from build123d import *

# Parameters (mm, degrees)
BOSS_EXTRUDE2_DEPTH = 5
SKETCH8_R           = 50
CUT_EXTRUDE6_DEPTH  = 20
SKETCH9_OUTSIDE_W   = 10.721
SKETCH9_OUTSIDE_H   = 17.86
SKETCH9_OUTSIDE_R   = 50
CUT_EXTRUDE7_DEPTH  = 20
SKETCH11_W          = 7
SKETCH11_H          = 2.5
BOSS_EXTRUDE4_DEPTH = 2
SKETCH12_OUTSIDE_W  = 9.685
SKETCH12_OUTSIDE_H  = 17.824
SKETCH12_OUTSIDE_R  = 50
CUT_EXTRUDE8_DEPTH  = 20
SKETCH13_R          = 0.3
CUT_EXTRUDE10_DEPTH = 21.130822139
SKETCH14_R          = 0.3
CUT_EXTRUDE11_DEPTH = 20
FILLET1_R           = 0.57


with BuildPart() as part:
    # Sketch1 → Boss-Extrude2 (new body)
    with BuildSketch(Plane.XY):
        Polygon((0, 0), (0, 8.5), (3, 8.5), (3, 2.5), (15, 2.5), (15, 8.5), (18, 8.5), (18, 0), (16, 0), (16, -3), (12.5, -2), (12.5, 0), (5.5, 0), (5.5, -2), (2, -3), (2, 0), align=None)
    extrude(amount=BOSS_EXTRUDE2_DEPTH)

    # Sketch8 → Cut-Extrude6 (cut)
    with BuildSketch(Plane(origin=(0, 0, 0), x_dir=(0, 0, -1), z_dir=(1, 0, 0))):
        with Locations((49, 2.5)):
            Circle(SKETCH8_R)
    extrude(amount=CUT_EXTRUDE6_DEPTH, mode=Mode.SUBTRACT)

    # Sketch9 outside → Cut-Extrude7 (cut)
    with BuildSketch(Plane(origin=(0, 0, 0), x_dir=(0, 0, -1), z_dir=(1, 0, 0))):
        with Locations((-2.8195, 2.75)):
            Rectangle(SKETCH9_OUTSIDE_W, SKETCH9_OUTSIDE_H)
        with Locations((47.1, 2.5)):
            Circle(SKETCH9_OUTSIDE_R, mode=Mode.SUBTRACT)
    extrude(amount=CUT_EXTRUDE7_DEPTH, mode=Mode.SUBTRACT)

    # Sketch11 → Boss-Extrude4 (add)
    with BuildSketch(Plane.XY.offset(4)):
        Polygon((0, 0), (0, 8.5), (3, 8.5), (3, 2.5), (2, 2.5), (2, 0), align=None)
        with Locations((9, 1.25)):
            Rectangle(SKETCH11_W, SKETCH11_H)
        Polygon((18, 8.5), (15, 8.5), (15, 2.5), (16, 2.5), (16, 0), (18, 0), align=None)
    extrude(amount=-BOSS_EXTRUDE4_DEPTH)

    # Sketch12 outside → Cut-Extrude8 (cut)
    with BuildSketch(Plane(origin=(0, 0, 0), x_dir=(0, 0, -1), z_dir=(1, 0, 0))):
        with Locations((-2.3195, 2.75)):
            Rectangle(SKETCH12_OUTSIDE_W, SKETCH12_OUTSIDE_H)
        with Locations((47, 2.5)):
            Circle(SKETCH12_OUTSIDE_R, mode=Mode.SUBTRACT)
    extrude(amount=CUT_EXTRUDE8_DEPTH, mode=Mode.SUBTRACT)

    # Sketch13 → Cut-Extrude10 (cut, through all)
    with BuildSketch(Plane(origin=(0, 0, 0), x_dir=(0, 0, -1), z_dir=(1, 0, 0))):
        with Locations(Location((-1.752335907, 7.52, 0), (0, 0, 270))):
            Circle(SKETCH13_R)
    extrude(amount=CUT_EXTRUDE10_DEPTH, mode=Mode.SUBTRACT)

    # Sketch14 → Cut-Extrude11 (cut)
    with BuildSketch(Plane(origin=(0, 0, 0), x_dir=(0, 0, -1), z_dir=(1, 0, 0))):
        with Locations(Location((-1.865607241, -1.2, 0), (0, 0, 270))):
            Circle(SKETCH14_R)
    extrude(amount=CUT_EXTRUDE11_DEPTH, mode=Mode.SUBTRACT)

    # Fillet1
    # the kernel refuses this fillet: 0.57 mm, written as the material it takes off along each edge
    with BuildSketch(Plane(origin=(4.276921505, 8.5, 2.638694584), x_dir=(0, 0, -1), z_dir=(-1, 0, 0)), Plane(origin=(19.276921505, 8.5, 2.638694584), x_dir=(0, 0, -1), z_dir=(-1, 0, 0))) as fillet1_piece_1:
        with BuildLine():
            CenterArc((0.507848876, 0.57), FILLET1_R, 186.30680233, 83.69319767)
            ThreePointArc((-0.058701439, 0.50738418), (-0.029998613, 0.253617132), (0, 0))
            Line((0, 0), (0.507848876, 0))
        make_face()
    extrude(amount=5.553843009, mode=Mode.SUBTRACT)
    with BuildSketch(Plane(origin=(2, 0, 2.937460889), x_dir=(0, 0.9990083494707687, 0.0445232263845563), z_dir=(-1, 0, 0))) as fillet1_piece_2:
        with BuildLine():
            CenterArc((0.545162753, 0.569991432), FILLET1_R, 182.551836528, 87.762310927)
            Line((-0.024272006, 0.544613193), (0, 0))
            ThreePointArc((0, 0), (0.274143997, -0.000751555), (0.548287995, 0))
        make_face()
    extrude(amount=3.370719987, mode=Mode.SUBTRACT)
    with BuildSketch(Plane(origin=(19.370719987, 0, 2.937460889), x_dir=(0, 0, -1), z_dir=(-1, 0, 0))) as fillet1_piece_3:
        with BuildLine():
            CenterArc((0.545153795, -0.57), FILLET1_R, 90, 87.762310927)
            ThreePointArc((-0.024411551, -0.547744285), (-0.012956585, -0.273838681), (0, 0))
            Line((0, 0), (0.545153795, 0))
        make_face()
    extrude(amount=3.370719987, mode=Mode.SUBTRACT)
    with BuildSketch(Plane(origin=(2, 0, 0.937460889), x_dir=(0, 0.9990278617443559, 0.04408323330360469), z_dir=(-1, 0, 0)), Plane(origin=(19.489241357, 0, 0.937460889), x_dir=(0, 0.9990278617443559, 0.04408323330360409), z_dir=(-1, 0, 0))) as fillet1_piece_4:
        with BuildLine():
            CenterArc((0.595706111, -0.569990001), FILLET1_R, 90.339381978, 92.187220026)
            Line((0.02626023, -0.595117444), (0, 0))
            ThreePointArc((0, 0), (0.296164915, -0.000877144), (0.592329831, 0))
        make_face()
    extrude(amount=3.489241357, mode=Mode.SUBTRACT)
    with BuildSketch(Plane(origin=(4.59733659, 8.5, 0.638694584), x_dir=(0, 0, 1), z_dir=(-1, 0, 0))) as fillet1_piece_5:
        with BuildLine():
            CenterArc((0.638934636, -0.57), FILLET1_R, 90, 96.164070516)
            ThreePointArc((0.072230095, -0.631204271), (0.037117605, -0.315487411), (0, 0))
            Line((0, 0), (0.638934636, 0))
        make_face()
    extrude(amount=6.194673181, mode=Mode.SUBTRACT)
    with BuildSketch(Plane(origin=(19.59733659, 8.5, 0.638694584), x_dir=(0, -0.993516243777255, 0.1136902517841086), z_dir=(-1, 0, 0))) as fillet1_piece_6:
        with BuildLine():
            CenterArc((0.638944899, 0.569988496), FILLET1_R, 173.471913452, 96.164070516)
            Line((0.07264064, 0.63479194), (0, 0))
            ThreePointArc((0, 0), (0.317661777, 0.0010091), (0.635323554, 0))
        make_face()
    extrude(amount=6.194673181, mode=Mode.SUBTRACT)


solid = part.part
Can you work these out from the model? Positions are in its coordinate system, mm. A direction names the side the tool comes from. Coordinates: 2 decimals unless noted, no trailing zeros. Order: outer loops, then holes, each group sorted by start corner. A loop starts at its lowest first (then second) coordinate and runs counter-clockwise, first axis right, second up. Notation, with made-up numbers: (9.25, 0.25) - (25.25, 0.25) arc R14 ccw to (25.25, 19.25) - close; hole circle Ø6 at (48, 44). An arc over 180 degrees is marked (long way). Answer as a JSON object with one key per item and string values. Group by question number.
Q1. Imagine slicing it at A-A (y = 2.75). Please give me the cut outline in (x, z), and give its area (3 significant figures).
Q2. We'd pull the mould along Y, two halves only. Please class faces 5 (the face through (9, 0, 2)), 6 (the face through (18, 4, 2)), 7 (the face through (8.874, 1.3, 0.986)), 8 (the face through (16.5, 8.5, 1.7)): +Y half, -Y half, draft (parallel to the pull), parting line (faces both ways), or undercut.
Q3. Will these pins go through, and if not, where does the flat tip stop? P1, Ø0.6, axis at y = -1, z = 1.5, coming from the +X side; P2, Ø0.9, axis at x = 1.5, z = 2, coming from the -Y side; P3, Ø0.6, axis at y = -0.5, z = 2, coming from the -X side; P4, Ø4, axis at x = 6.5, y = 3, coming from the +Z side.
Q4. Imagine slicing it at C-C (x = 15.75). Please give me the cut outline in (y, z), and give its area (3 significant figures).
Q5. On a 3-axis mill with a long thin cutter (end or side, diameter ignored), from which of +Z, -Z, +X, -X, +Y, -Y can I reach the whole of each face in a straight line? I mean faces 1 (the face through (14.275, -2.507, 1.683)), 2 (the face through (3.726, -0.216, 2.826)), 3 (the face through (1.479, 4.327, 2.967)), 4 (the face through (17, 0, 2)). Say none if no direction works.
Q6. Imagine slicing it at B-B (y = 7.52). Please give me the cut outline in (x, z).
Q7. I need wall thicknesses on line 1 (X direction, y = -0.75, z = 1.9); line 2 (X direction, y = 4.25, z = 1.25); line 3 (Y direction, x = 11.75, z = 1.4). Which ranges of each line are inside material? Lowest first, please. Write a range as from..to.
Q8. Imagine slicing it at D-D (x = 1.5). Please give me the cut outline in (y, z).
Determined:
{
 "1": {"outline": "(0, 1) - (3, 1) - (3, 3) - (0, 3) - close; (15, 1) - (18, 1) - (18, 3) - (15, 3) - close", "area": "12.0 mm2"},
 "2": {"face 5": "-Y half", "face 6": "draft", "face 7": "undercut", "face 8": "+Y half"},
 "3": {"P1": "stops at x = 16", "P2": "stops at y = 0", "P3": "stops at x = 2", "P4": "stops at z = 3"},
 "4": {"outline": "(-2.93, 0.7) arc R50 cw to (7.87, 0.71) arc R0.57 ccw to (8.5, 1.28) - (8.5, 2.13) arc R0.57 ccw to (7.99, 2.7) arc R50 ccw to (2.5, 3) - (2.5, 2.9) arc R50 ccw to (-2.93, 2.6) - close; hole circle Ø0.6 at (-1.2, 1.87); hole circle Ø0.6 at (7.52, 1.75)", "area": "21.6 mm2"},
 "5": {"face 1": "+Z, -Z, -Y", "face 2": "+Z, -Y", "face 3": "+Z, +X, -X", "face 4": "+Z, -Z, +X, -Y"},
 "6": {"outline": "(0, 0.75) - (3, 0.75) - (3, 1.45) - (0, 1.45) - close; (0, 2.05) - (3, 2.05) - (3, 2.75) - (0, 2.75) - close; (15, 0.75) - (18, 0.75) - (18, 1.45) - (15, 1.45) - close; (15, 2.05) - (18, 2.05) - (18, 2.75) - (15, 2.75) - close"},
 "7": {"line 1": "x = 2..5.5, 12.5..16", "line 2": "x = 0..3, 15..18", "line 3": "y = 0..2.5"},
 "8": {"outline": "(0, 1.53) arc R0.57 ccw to (0.59, 0.96) arc R50 cw to (7.87, 0.71) arc R0.57 ccw to (8.5, 1.28) - (8.5, 2.13) arc R0.57 ccw to (7.99, 2.7) arc R50 ccw to (0.55, 2.96) arc R0.57 ccw to (0, 2.39) - close; hole circle Ø0.6 at (7.52, 1.75)"}
}
